```python
from build123d import *

# Parameters (mm, degrees)
SKETCH1_W                                            = 16.1
SKETCH1_H                                            = 14.1
BOSS_EXTRUDE1_DEPTH                                  = 7
SKETCH3_W                                            = 12.1
SKETCH3_H                                            = 10.1
CUT_EXTRUDE1_DEPTH                                   = 4
CSK_FOR_M1_6_COUNTERSUNK_FLAT_HEAD_SCREW_D           = 2
CSK_FOR_M1_6_COUNTERSUNK_FLAT_HEAD_SCREW_DEPTH       = 3
CSK_FOR_M1_6_COUNTERSUNK_FLAT_HEAD_SCREW_CSINK_D     = 4
CSK_FOR_M1_6_COUNTERSUNK_FLAT_HEAD_SCREW_CSINK_ANGLE = 90
SKETCH8_R                                            = 2
CUT_EXTRUDE2_DEPTH                                   = 4
FILLET1_R                                            = 2
FILLET2_R                                            = 0.2


with BuildPart() as part:
    # Sketch1 → Boss-Extrude1 (new body)
    with BuildSketch(Plane(origin=(0, 0, 0), x_dir=(1, 0, 0), z_dir=(0, 1, 0))):
        Rectangle(SKETCH1_W, SKETCH1_H)
    extrude(amount=BOSS_EXTRUDE1_DEPTH)

    # Sketch3 → Cut-Extrude1 (cut)
    with BuildSketch(Plane(origin=(0, 7, 0), x_dir=(1, 0, 0), z_dir=(0, 1, 0))):
        Rectangle(SKETCH3_W, SKETCH3_H)
    extrude(amount=-CUT_EXTRUDE1_DEPTH, mode=Mode.SUBTRACT)

    # CSK for M1.6 Countersunk Flat Head Screw1
    with Locations(Plane(origin=(0, 0, 0), x_dir=(-1, 0, 0), z_dir=(0, -1, 0))):
        with Locations((4.5, 0), (-4.5, 0)):
            CounterSinkHole(CSK_FOR_M1_6_COUNTERSUNK_FLAT_HEAD_SCREW_D / 2, CSK_FOR_M1_6_COUNTERSUNK_FLAT_HEAD_SCREW_CSINK_D / 2, depth=CSK_FOR_M1_6_COUNTERSUNK_FLAT_HEAD_SCREW_DEPTH, counter_sink_angle=CSK_FOR_M1_6_COUNTERSUNK_FLAT_HEAD_SCREW_CSINK_ANGLE)

    # Sketch8 → Cut-Extrude2 (cut, through all)
    with BuildSketch(Plane(origin=(0, 3, 0), x_dir=(1, 0, 0), z_dir=(0, 1, 0))):
        Circle(SKETCH8_R)
    extrude(amount=-CUT_EXTRUDE2_DEPTH, mode=Mode.SUBTRACT)

    # Fillet1
    fillet1_edges = [part.edges().sort_by_distance(p)[0] for p in [
        (-8.05, 3.5, -7.05),
        (8.05, 3.5, -7.05),
        (8.05, 3.5, 7.05),
        (-8.05, 3.5, 7.05),
    ]]
    fillet(fillet1_edges, radius=FILLET1_R)

    # Fillet2
    fillet2_edges = [part.edges().sort_by_distance(p)[0] for p in [
        (-6.05, 5, 5.05),
        (-6.05, 5, -5.05),
        (6.05, 5, -5.05),
        (6.05, 5, 5.05),
    ]]
    fillet(fillet2_edges, radius=FILLET2_R)


solid = part.part
```
The model under review builds one solid part; all positions refer to its coordinate system, in mm. A direction names the side the tool comes from. Give positions to 0.01 mm unless a question says otherwise; leave off trailing zeros. Write each loop counter-clockwise with the first axis right and the second up, starting at its lowest first coordinate (ties: lowest second). Pieces come first, ordered by that corner, then holes.
(1) Consider section A-A, the plane y = 2.25. Give the boundary of the cut face in (x, z), and give its area (3 significant figures).
(2) To check wall thickness, follow L1, parallel to Z at x = 4.5, y = 2.5; L2, parallel to Z at x = -5.5, y = 4.75; L3, parallel to X at y = 5.25, z = 0.5. State the ranges of each line that lie inside material, in increasing order.
(3) For P1, Ø4.5, axis at x = 0, z = 0, coming from the +Y side; P2, Ø2.5, axis at x = 4.5, z = 0, coming from the -Y side; P3, Ø1.5, axis at x = 5, z = -1, coming from the -Y side, all flat-tipped, find the tip position at first contact; note any pin that passes through.
(4) The part is to be moulded in two halves that separate along X. For faces 3 (the flat face through (2, 0, -2)), 4 (the cylindrical face through (0, 2, 2)), 5 (the cylindrical face through (-7.48, 3.55, -6.45)), say which applies: released by +X, released by -X, zero draft, split by the parting line, or undercut.
(5) Consider section D-D, the plane z = 0. Give the boundary of the cut face in (x, y).
(6) Tool access review of faces 1 (the flat face through (0, 5, -5.05)), 2 (the flat face through (0, 7, 6)): name each direction out of +Z, -Z, +X, -X, +Y, -Y from which nothing blocks a thin tool from reaching the whole face with its end or side.
(7) Consider section B-B, the plane x = -4.5. Give the boundary of the cut face in (y, z), and give its area (3 significant figures).
(8) Consider section C-C, the plane z = -4. Give the boundary of the cut face in (x, y), and give its area (3 significant figures).
Returned:
1. outline: (-8.05, -5.05) arc R2 ccw to (-6.05, -7.05) - (6.05, -7.05) arc R2 ccw to (8.05, -5.05) - (8.05, 5.05) arc R2 ccw to (6.05, 7.05) - (-6.05, 7.05) arc R2 ccw to (-8.05, 5.05) - close; hole circle Ø2 at (-4.5, 0); hole circle Ø4 at (0, 0); hole circle Ø2 at (4.5, 0)
1. area: 205 mm2
2. L1: z = -7.05 to -1, 1 to 7.05
2. L2: z = -7.05 to -5.05, 5.05 to 7.05
2. L3: x = -8.05 to -6.05, 6.05 to 8.05
3. P1: stops at y = 3
3. P2: stops at y = 0.75
3. P3: stops at y = 0.13
4. face 3: zero draft
4. face 4: undercut
4. face 5: released by -X
5. outline: (-8.05, 0) - (-6.5, 0) - (-5.5, 1) - (-5.5, 3) - (-6.05, 3) - (-6.05, 7) - (-8.05, 7) - close; (-3.5, 1) - (-2.5, 0) - (-2, 0) - (-2, 3) - (-3.5, 3) - close; (2, 0) - (2.5, 0) - (3.5, 1) - (3.5, 3) - (2, 3) - close; (5.5, 1) - (6.5, 0) - (8.05, 0) - (8.05, 7) - (6.05, 7) - (6.05, 3) - (5.5, 3) - close
6. face 1: +Y
6. face 2: +Z, -Z, +X, -X, +Y
7. outline: (0, -7.05) - (7, -7.05) - (7, -5.05) - (3, -5.05) - (3, -1) - (1, -1) - (0, -2) - close; (0, 2) - (1, 1) - (3, 1) - (3, 5.05) - (7, 5.05) - (7, 7.05) - (0, 7.05) - close
7. area: 51.3 mm2
8. outline: (-8.05, 0) - (8.05, 0) - (8.05, 7) - (6.05, 7) - (6.05, 3) - (-6.05, 3) - (-6.05, 7) - (-8.05, 7) - close
8. area: 64.3 mm2
